Part model, mm, in its own coordinate system. Give positions to 0.01 mm unless a question says otherwise; leave off trailing zeros. Write each loop counter-clockwise with the first axis right and the second up, starting at its lowest first coordinate (ties: lowest second). Pieces come first, ordered by that corner, then holes.
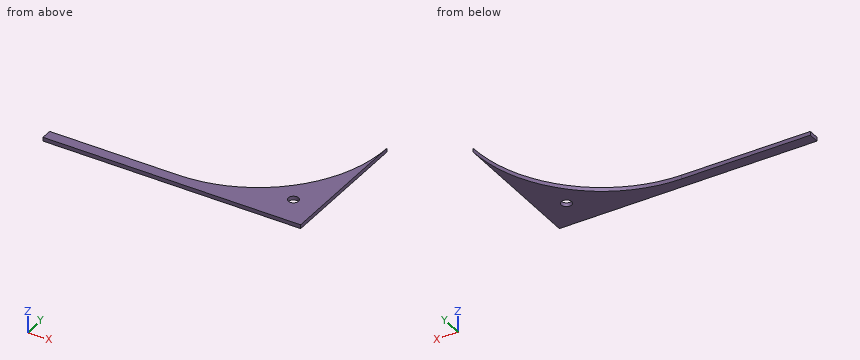
Autodesk Inventor part; units mm, degrees
ref_plane "YZ Plane" through (0, 0, 0) normal (1, 0, 0) x (0, 1, 0)
ref_plane "XZ Plane" through (0, 0, 0) normal (0, 1, 0) x (-1, 0, 0)
ref_plane "XY Plane" through (0, 0, 0) normal (0, 0, 1) x (1, 0, 0)
sketch "草圖1" plane through (0, 0, 0) normal (0, 0, 1) x (1, 0, 0)
  line L0 (0, -80) -> (100, -80)
  arc A0 (100, -80) -> (200, 20) centre (100, 20) ccw
  line L1 (200, 20) -> (200, 40)
  line L2 (200, 40) -> (100, 40)
  line L3 (100, 40) -> (100, -80)
  line L4 (100, -80) -> (200, -80)
  line L5 (200, -80) -> (200, 40)
  line L6 (215, -80) -> (200, -80)
  circle A1 centre (180, -65) radius 4
  line L7 (200, -80) -> (0, -80)
  line L8 (0, -80) -> (0, -88.525)
  line L9 (0, -88.525) -> (200, -88.525)
  line L10 (200, -88.525) -> (200, -80)
  point P0 (200, 20)
  dimension "d5" = 8
  dimension "d6" = 8.525
  dimension "d12" = 15
  dimension "d13" = 20
extrude "擠出1" add sketch "草圖1" along normal blind 3 contours L0 L4 L10 L9 L8 | A0 L5 L4
sketch "草圖3" plane through (0, 0, 3) normal (0, 0, 1) x (1, 0, 0)
  line L0 (200, -88.525) -> (200, 20)
  line L1 (0, -88.525) -> (200, -88.525)
  line L2 (0, -88.525) -> (200, -88.525)
  line L3 (200, -88.525) -> (200, -88.375)
  line L4 (200, -88.375) -> (0, -88.375)
  line L5 (0, -88.375) -> (0, -88.525)
  point P0 (0, 0)
  dimension "d11" = 0.15
extrude "擠出2" cut sketch "草圖3" against normal up to surface (3 mm away)
1) Saw through at D-D, the plane x = 29. Write the cut outline in (y, z) (3 decimals), then the cut area to 3 significant figures.
Answers follow:
outline: (-88.375, 0) - (-80, 0) - (-80, 3) - (-88.375, 3) - close
area: 25.1 mm2
2) Wall check: L1, parallel to Y at x = 180, z = 1.5 (3 decimals); L2, parallel to Y at x = 82.5, z = 1.1 (3 decimals); L3, parallel to X at y = -64.5, z = 1.35. Give the ranges that are in metal, low to high.
Answers follow:
L1: y = -88.375 to -69, -61 to -40
L2: y = -88.375 to -80
L3: x = 153.48 to 176.03, 183.97 to 200
3) Saw through at C-C, the plane x = 180. Write the cut outline in (y, z) (3 decimals), then the cut area to 3 significant figures.
Answers follow:
outline: (-88.375, 0) - (-69, 0) - (-69, 3) - (-88.375, 3) - close; (-61, 0) - (-40, 0) - (-40, 3) - (-61, 3) - close
area: 121 mm2
4) Saw through at B-B, the plane y = -65. Write the cut outline in (x, z).
Answers follow:
outline: (152.68, 0) - (176, 0) - (176, 3) - (152.68, 3) - close; (184, 0) - (200, 0) - (200, 3) - (184, 3) - close
5) Pin check, flat tips, straight feed: pin 1 Ø1.5 at (x, z) = (153.5, 1) entering from +Y; pin 2 Ø1.5 at (y, z) = (6, 1.5) entering from -X; pin 3 Ø9 at (x, y) = (180, -65) entering from +Z. Stop position of each tip, or through.
Answers follow:
pin 1: stops at y = -64.01
pin 2: stops at x = 198.91
pin 3: stops at z = 3
6) Saw through at A-A, the plane z = 0.8. Write the cut outline in (x, y) (3 decimals), then the cut area to 3 significant figures.
Answers follow:
outline: (0, -88.375) - (200, -88.375) - (200, 20) arc R100 cw to (100, -80) - (0, -80) - close; hole circle Ø8 at (180, -65)
area: 3,770 mm2
